from build123d import *

# Parameters (mm, degrees)
CROQUIS3_R              = 6
SALIENTE_EXTRUIR1_DEPTH = 4.5
MATRIZC2_COUNT          = 4
CROQUIS4_R              = 4
CORTAR_EXTRUIR1_DEPTH   = 9
REDONDEO1_R             = 1


with BuildPart() as part:
    # Croquis1 → Recubrir2 section 0
    with BuildSketch(Plane(origin=(0, 0, 0), x_dir=(0, 0, -1), z_dir=(1, 0, 0))):
        Polygon((2.828427125, -4.242640687), (-4.242640687, 2.828427125), (-2.828427125, 4.242640687), (4.242640687, -2.828427125), align=None)
    # Croquis2 → Recubrir2 section 1
    with BuildSketch(Plane(origin=(21, 0, 0), x_dir=(0, 0, -1), z_dir=(1, 0, 0))):
        Polygon((4.242640687, -2.828427125), (-2.828427125, 4.242640687), (-4.242640687, 2.828427125), (2.828427125, -4.242640687), align=None)
    recubrir2 = loft()

    # Croquis3 → Saliente-Extruir1 (add, symmetric)
    with BuildSketch(Plane(origin=(0, 0, 0), x_dir=(1, 0, 0), z_dir=(0, 1, 0))):
        with Locations((-4, 0)):
            Circle(CROQUIS3_R)
    extrude(amount=SALIENTE_EXTRUIR1_DEPTH, both=True)

    # MatrizC2: Recubrir2 ×4 about axis
    matrizc2_axis = Axis((-4, 0, 0), (0, 1, 0))
    for i in range(1, MATRIZC2_COUNT):
        add(recubrir2.rotate(matrizc2_axis, i * 360 / MATRIZC2_COUNT))

    # Croquis4 → Cortar-Extruir1 (cut)
    with BuildSketch(Plane(origin=(0, 4.5, 0), x_dir=(1, 0, 0), z_dir=(0, 1, 0))):
        with Locations((-4, 0)):
            Circle(CROQUIS4_R)
    extrude(amount=-CORTAR_EXTRUIR1_DEPTH, mode=Mode.SUBTRACT)

    # Redondeo1
    redondeo1_edges = [part.edges().sort_by_distance(p)[0] for p in [
        (-7.535533906, 3.535533906, 25),
        (-0.464466094, -3.535533906, 25),
        (-29, -3.535533906, 3.535533906),
        (-29, 3.535533906, -3.535533906),
        (-7.535533906, -3.535533906, -25),
        (-0.464466094, 3.535533906, -25),
        (21, -3.535533906, -3.535533906),
        (21, 3.535533906, 3.535533906),
    ]]
    fillet(redondeo1_edges, radius=REDONDEO1_R)


solid = part.part
Could you check a few things on this model? Use its own coordinates, in mm. A direction names the side the tool comes from. Give positions to 0.01 mm unless a question says otherwise; leave off trailing zeros. Order: outer loops, then holes, each group sorted by start corner. A loop starts at its lowest first (then second) coordinate and runs counter-clockwise, first axis right, second up. Notation, with made-up numbers: (88, 30.25) - (145, 30.25) arc R15 ccw to (145, 43.25) - close; hole circle Ø7 at (-17.5, -37.5). An arc over 180 degrees is marked (long way). One line per item, written item: value. Start each with the question number.
1. For P1, Ø5, axis at y = -1, z = -16.5, coming from the -X side; P2, Ø5, axis at x = -11.5, y = -2, coming from the -Z side; P3, Ø6, axis at x = -23, z = 4, coming from the +Y side, each with a flat end and sliding along its axis, tell me the tip position at first contact or that it passes through.
2. If I drill on probe 1 along X at (y, z) = (1.5, 0); probe 2 along X at (y, z) = (-0.75, 0); probe 3 along Z at (x, y) = (-4, 0.75), over which ranges is the centre line in solid material (lowest first)?
3. For faces 1 (the face through (-0.455, 3.526, -14.26)), 2 (the face through (-7.545, -3.526, -14.26)), 3 (the face through (-8.42, 0.06, -4.06)), 4 (the face through (-7.545, 3.526, 14.26)), which set-ups out of +Z, -Z, +X, -X, +Y, -Y let a thin tool reach every point of the face, with its end or its side?
4. Imagine slicing it at D-D on z = 9. List the corners of the cut face in (x, y) for me.
5. Imagine slicing it at C-C on x = -21.5. List the corners of the cut face in (y, z) for me, plus the area to 3 significant figures.
6. Imagine slicing it at A-A on x = -4. List the corners of the cut face in (y, z) for me.
7. Imagine slicing it at B-B on z = 0. List the corners of the cut face in (x, y) for me.
Values:
1. P1: x = -8.24
1. P2: z = -3.32
1. P3: y = 0.41
2. probe 1: -10 to -8, 0 to 2
2. probe 2: -29 to -8, 0 to 21
2. probe 3: -25 to -4, 4 to 25
3. face 1: -Z, +X, +Y
3. face 2: -Z, -X, -Y
3. face 3: none
3. face 4: +Z, -X, +Y
4. outline: (-8.24, 2.83) - (-1.17, -4.24) - (0.24, -2.83) - (-6.83, 4.24) - close
5. outline: (-4.24, 2.83) - (2.83, -4.24) - (4.24, -2.83) - (-2.83, 4.24) - close
5. area: 20.0 mm²
6. outline: (-4.5, -6) - (-1.41, -6) - (-1.41, -25) - (1.41, -25) - (1.41, -6) - (4.5, -6) - (4.5, -4) - (-4.5, -4) - close; (-4.5, 4) - (4.5, 4) - (4.5, 6) - (1.41, 6) - (1.41, 25) - (-1.41, 25) - (-1.41, 6) - (-4.5, 6) - close
7. outline: (-29, -1.41) - (-10, -1.41) - (-10, -4.5) - (-8, -4.5) - (-8, 4.5) - (-10, 4.5) - (-10, 1.41) - (-29, 1.41) - close; (0, -4.5) - (2, -4.5) - (2, -1.41) - (21, -1.41) - (21, 1.41) - (2, 1.41) - (2, 4.5) - (0, 4.5) - close
